Input: part model. Units: mm. Frame: model coordinates. A direction names the side the tool comes from. Coordinates: 2 decimals unless noted, no trailing zeros. Order: outer loops, then holes, each group sorted by start corner. A loop starts at its lowest first (then second) coordinate and runs counter-clockwise, first axis right, second up. Notation, with made-up numbers: (-35, -17) - (-5, -17) arc R18 ccw to (-5, -12) - close; hole circle Ø8 at (39.5, -24.5). An arc over 180 degrees is marked (long way). Answer as CSV lines item,"result". Start each with the question number.
Item 1: First-contact query: pin 1 (2 mm diameter, centred on y = 2.5, z = -1.5, fed in from +X); pin 2 (0.6 mm diameter, centred on y = 3, z = 0, fed in from +X); pin 3 (0.6 mm diameter, centred on x = 0, y = -1, fed in from -Z). Flat tips, straight axial feed; report the tip coordinate or a pass-through.
Item 2: Material intervals for line 1 along X through (y, z) = (-1.5, 0.05); line 2 along Z through (x, y) = (1.9, -2.75); line 3 along Y through (x, z) = (-1.1, -1.55), sorted ascending.
Item 3: Section B-B (x = 0). Output: boundary loops of the cut face in (y, z), and give its area (3 significant figures).
Item 4: Section C-C (z = -0.45). Output: boundary loops of the cut face in (x, y).
Item 5: Access query for faces 1 (the flat face through (2, 1, -0.25)), 2 (the cylindrical face through (-1.5, 6.2, -0.07)), 3 (the flat face through (-2, 0, 0.25)). Directions: +Z, -Z, +X, -X, +Y, -Y. A direction counts if a zero-diameter tool reaches every point of the face in a straight line with its end or side. Return the directions, or none.
Item 6: Section D-D (x = -1.25). Output: boundary loops of the cut face in (y, z), and give its area (3 significant figures).
Item 7: Section A-A (y = -0.5). Output: boundary loops of the cut face in (x, z), and give its area (3 significant figures).
from build123d import *

# Parameters (mm, degrees)
ESBO_O1_W                       = 0.5
ESBO_O1_H                       = 0.5
RESSALTO_EXTRUS_O1_DEPTH        = 1
RESSALTO_EXTRUS_O1_DEPTH_BACK   = 4
RESSALTO_EXTRUS_O1_2_DEPTH      = 1
RESSALTO_EXTRUS_O1_2_DEPTH_BACK = 4
RESSALTO_EXTRUS_O1_3_DEPTH      = 1
RESSALTO_EXTRUS_O1_3_DEPTH_BACK = 4
ESBO_O2_W                       = 0.5
ESBO_O2_H                       = 2.43
RESSALTO_EXTRUS_O2_DEPTH        = 0.5
RESSALTO_EXTRUS_O3_DEPTH        = 1


with BuildPart() as part:
    # Esbo_o1 → Ressalto-extrus_o1 (new body, two sides)
    with BuildSketch(Plane(origin=(0, 0, 0), x_dir=(1, 0, 0), z_dir=(0, 1, 0))) as ressalto_extrus_o1_sk:
        Rectangle(ESBO_O1_W, ESBO_O1_H)
    extrude(amount=RESSALTO_EXTRUS_O1_DEPTH)
    extrude(ressalto_extrus_o1_sk.sketch, amount=-RESSALTO_EXTRUS_O1_DEPTH_BACK)



with BuildPart() as body_2:
    # Esbo_o1 → Ressalto-extrus_o1 2 (new body, two sides)
    with BuildSketch(Plane(origin=(0, 0, 0), x_dir=(1, 0, 0), z_dir=(0, 1, 0))) as ressalto_extrus_o1_2_sk:
        with Locations((2, 0)):
            Rectangle(ESBO_O1_W, ESBO_O1_H)
    extrude(amount=RESSALTO_EXTRUS_O1_2_DEPTH)
    extrude(ressalto_extrus_o1_2_sk.sketch, amount=-RESSALTO_EXTRUS_O1_2_DEPTH_BACK)


with BuildPart() as body_3:
    # Esbo_o1 → Ressalto-extrus_o1 3 (new body, two sides)
    with BuildSketch(Plane(origin=(0, 0, 0), x_dir=(1, 0, 0), z_dir=(0, 1, 0))) as ressalto_extrus_o1_3_sk:
        with Locations((-2, 0)):
            Rectangle(ESBO_O1_W, ESBO_O1_H)
    extrude(amount=RESSALTO_EXTRUS_O1_3_DEPTH)
    extrude(ressalto_extrus_o1_3_sk.sketch, amount=-RESSALTO_EXTRUS_O1_3_DEPTH_BACK)


with BuildPart() as part_1:
    add(part.part)

    add(body_2.part)  # Ressalto-extrus_o2 merges body 2

    add(body_3.part)  # Ressalto-extrus_o2 merges body 3
    # Esbo_o2 → Ressalto-extrus_o2 (add)
    with BuildSketch(Plane.XY.offset(0.25)):
        with BuildLine():
            Line((-2.25, 2.2), (-2.25, 1))
            Line((-2.25, 1), (-1.75, 1))
            Line((-1.75, 1), (-1.75, 1.8))
            ThreePointArc((-1.75, 1.8), (-1.691421356, 1.941421356), (-1.55, 2))
            Line((-1.55, 2), (-0.867667764, 2))
            ThreePointArc((-0.867667764, 2), (-0.726246408, 2.058578644), (-0.667667764, 2.2))
            Line((-0.667667764, 2.2), (-0.667667764, 2.376879859))
            Line((-0.667667764, 2.376879859), (-0.55, 2.479277604))
            Line((-0.55, 2.479277604), (-0.55, 3.43))
            Line((-0.55, 3.43), (-1.05, 3.43))
            Line((-1.05, 3.43), (-1.05, 2.83866396))
            Line((-1.05, 2.83866396), (-2.25, 2.2))
        make_face()
        with Locations((0, 2.215)):
            Rectangle(ESBO_O2_W, ESBO_O2_H)
        with BuildLine():
            Line((1.75, 1), (1.75, 1.8))
            ThreePointArc((1.75, 1.8), (1.691421356, 1.941421356), (1.55, 2))
            Line((1.55, 2), (0.75, 2))
            ThreePointArc((0.75, 2), (0.608578644, 2.058578644), (0.55, 2.2))
            Line((0.55, 2.2), (0.55, 3.43))
            Line((0.55, 3.43), (1.05, 3.43))
            Line((1.05, 3.43), (1.05, 2.83866396))
            Line((1.05, 2.83866396), (2.25, 2.2))
            Line((2.25, 2.2), (2.25, 1))
            Line((2.25, 1), (1.75, 1))
        make_face()
    extrude(amount=-RESSALTO_EXTRUS_O2_DEPTH)

    # Esbo_o3 → Ressalto-extrus_o3 (add)
    with BuildSketch(Plane(origin=(0, 3.43, 0), x_dir=(1, 0, 0), z_dir=(0, 1, 0))):
        with BuildLine():
            Line((1.5, 1.322875656), (1.5, -1.322875656))
            ThreePointArc((1.5, -1.322875656), (-2, 0), (1.5, 1.322875656))
        make_face()
    extrude(amount=RESSALTO_EXTRUS_O3_DEPTH)

    # Esbo_o4 → Revolu_o1 (revolve)
    with BuildSketch(Plane.XY):
        with BuildLine():
            Line((0, 4.43), (1.5, 4.43))
            Line((1.5, 4.43), (1.5, 7.93))
            ThreePointArc((1.5, 7.93), (1.060660172, 8.990660172), (0, 9.43))
            Line((0, 9.43), (0, 4.43))
        make_face()
    revolve(axis=Axis((0, 4.43, 0), (0, 1, 0)))


solid = part_1.part
Determined:
1,pin 1,"stops at x = 1.5"
1,pin 2,"stops at x = 1.31"
1,pin 3,"stops at z = -0.25"
2,line 1,"x = -2.25 to -1.75, -0.25 to 0.25, 1.75 to 2.25"
2,line 2,"z = -0.25 to 0.25"
2,line 3,"y = 3.43 to 4.43"
3,outline,"(-4, -0.25) - (3.43, -0.25) - (3.43, -2) - (4.43, -2) - (4.43, -1.5) - (7.93, -1.5) arc R1.5 ccw to (7.93, 1.5) - (4.43, 1.5) - (4.43, 2) - (3.43, 2) - (3.43, 0.25) - (-4, 0.25) - close"
3,area,"21.7 mm^2"
4,outline,"(-1.95, 3.43) - (1.5, 3.43) - (1.5, 4.43) - (1.43, 4.43) - (1.43, 7.93) arc R1.43 ccw to (-1.43, 7.93) - (-1.43, 4.43) - (-1.95, 4.43) - close"
5,face 1,"-Z, +X, -X, -Y"
5,face 2,"+Y"
5,face 3,"+Z, +X, -X, -Y"
6,outline,"(2, -0.25) - (2.73, -0.25) - (2.73, 0.25) - (2, 0.25) - close; (3.43, -1.56) - (4.43, -1.56) - (4.43, -0.83) - (7.93, -0.83) arc R0.83 ccw to (7.93, 0.83) - (4.43, 0.83) - (4.43, 1.56) - (3.43, 1.56) - close"
6,area,"10.4 mm^2"
7,outline,"(-2.25, -0.25) - (-1.75, -0.25) - (-1.75, 0.25) - (-2.25, 0.25) - close; (-0.25, -0.25) - (0.25, -0.25) - (0.25, 0.25) - (-0.25, 0.25) - close; (1.75, -0.25) - (2.25, -0.25) - (2.25, 0.25) - (1.75, 0.25) - close"
7,area,"0.750 mm^2"
